The listing builds one solid part. Answer for the finished solid, in the listing's coordinates (mm). A direction names the side the tool comes from. Coordinates: 2 decimals unless noted, no trailing zeros. Loops run counter-clockwise (first coordinate to the right, second up) from the corner with the lowest first, then second, coordinate; pieces in that order, holes last. Notation, with made-up numbers: (-22, 77.25) -> (-11, 77.25) arc R12 ccw to (-11, 87.25) -> close; hole circle Ø4 at (-9, 81.25). An arc over 180 degrees is marked (long way). Answer in a Markdown table with one row per item.
Autodesk Inventor part; units mm, degrees
ref_plane "YZ Plane" through (0, 0, 0) normal (1, 0, 0) x (0, 1, 0)
ref_plane "XZ Plane" through (0, 0, 0) normal (0, 1, 0) x (-1, 0, 0)
ref_plane "XY Plane" through (0, 0, 0) normal (0, 0, 1) x (1, 0, 0)
sketch "Sketch1" plane through (0, 0, 0) normal (0, 1, 0) x (-1, 0, 0)
  line L0 (0, 0) -> (2.5, 0)
  line L1 (2.5, 0) -> (2.5, -25)
  line L2 (2.5, -25) -> (0, -25)
  line L3 (0, -25) -> (0, 0)
  line L4 (0, -25) -> (2.775, -25)
  line L5 (0, -26.3) -> (2.85, -26.3)
  line L6 (2.85, -26.3) -> (1.55, -25)
  line L7 (2.85, -26.3) -> (4.6885, -26.3) construction
  line L8 (0, -26.3) -> (0, -25)
  dimension "d1" = 25
  dimension "d2" = 2.775
  dimension "d20" = 2.85
  dimension "d21" = 1.3
  dimension "d22" = 135
revolve "Revolution1" add sketch "Sketch1" angle 360 about axis through (0, 0, -25) along (0, 0, 1)
sketch "Sketch4" plane through (0, 0, -26.3) normal (0, 0, -1) x (-1, 0, 0)
  circle A0 centre (0, 0) radius 1.55
  line L0 (0, 1.1547) -> (1, 0.5774)
  line L1 (1, 0.5774) -> (1, -0.5774)
  line L2 (1, -0.5774) -> (0, -1.1547)
  line L3 (0, -1.1547) -> (-1, -0.5774)
  line L4 (-1, -0.5774) -> (-1, 0.5774)
  line L5 (-1, 0.5774) -> (0, 1.1547)
  dimension "d23" = 2
extrude "Extrusion2" cut sketch "Sketch4" against normal blind 1.2 contours L0 L1 L2 L3 L4 L5
properties part number "m3 spacer bolt combo"
Item 1: A tool of negligible diameter and unlimited length cuts with its end or side. For faces 4 (the face through (-2, 0, -25)), 5 (the face through (-1.2, 0, -26.3)), 6 (the face through (0.51, 0.86, -25.71)), from which of +Z, -Z, +X, -X, +Y, -Y can it reach the whole face along a straight path? Write none if from no direction.
Findings below:
| item | result |
|---|---|
| face 4 | none |
| face 5 | -Z, +X, -X, +Y, -Y |
| face 6 | -Z |
Item 2: Flat-ended cylindrical pins translate along their axes: pin 1 Ø1 at (x, y) = (0, 0) entering from -Z; pin 2 Ø1 at (x, z) = (-0.5, -4.5) entering from +Y; pin 3 Ø1 at (x, z) = (-1, -13) entering from -Y. Find the tip coordinate at first contact, or state that the pin passes through.
Findings below:
| item | result |
|---|---|
| pin 1 | stops at z = -25.1 |
| pin 2 | stops at y = 2.5 |
| pin 3 | stops at y = -2.45 |
Item 3: Determine the mould class of faces 1 (the face through (0.54, -2.44, -12.68)), 2 (the face through (0, 0, 0)), 3 (the face through (-1, 0, -26)) for opening direction Y: +Y half, -Y half, draft (parallel to the pull), parting line (faces both ways), or undercut.
Findings below:
| item | result |
|---|---|
| face 1 | parting line |
| face 2 | draft |
| face 3 | undercut |
Item 4: A cutting plane is placed at A-A, the plane y = 0. Determine the outline of the cut face in (x, z).
Findings below:
| item | result |
|---|---|
| outline | (-2.85, -26.3) -> (-1, -26.3) -> (-1, -25.1) -> (1, -25.1) -> (1, -26.3) -> (2.85, -26.3) -> (1.55, -25) -> (2.5, -25) -> (2.5, 0) -> (-2.5, 0) -> (-2.5, -25) -> (-1.55, -25) -> close |
Item 5: A cutting plane is placed at B-B, the plane z = -18. Determine the outline of the cut face in (x, y).
Findings below:
| item | result |
|---|---|
| outline | circle Ø5 at (0, 0) |
Item 6: Find the intervals of material crossed by probe 1 along Z at (x, y) = (-0.9, -0.25); probe 2 along Z at (x, y) = (-1.35, -2); probe 3 along Z at (x, y) = (0.1, -2), in increasing order.
Findings below:
| item | result |
|---|---|
| probe 1 | z = -25.1 to 0 |
| probe 2 | z = -26.3 to -25.86, -25 to 0 |
| probe 3 | z = -26.3 to -25.45, -25 to 0 |
